Geometry: final body of the model. Coordinates: model frame, mm. A direction names the side the tool comes from. Round coordinates to 2 decimals unless told otherwise and drop trailing zeros. Write each loop counter-clockwise with the first axis right and the second up, starting at its lowest first coordinate (ties: lowest second). Pieces come first, ordered by that corner, then holes. Notation, with made-up numbers: M 33,-24.75 L 81,-24.75 A12 ccw 81,-14.75 Z; hole C -1.75,-10.75 d5. An arc over 180 degrees is marked long. Put each result on its own line as item: value. Start each with the question number.
```python
from build123d import *

# Parameters (mm, degrees)
F0_W      = 80
F0_H      = 17
F0_R      = 1.05
F1_DEPTH  = 2.5
F3_DEPTH  = 43
F5_DEPTH  = 25
F7_D      = 3.3
F8_D      = 3.3
F4_R      = 4.5
F9_DEPTH  = 4.0010001
F10_R     = 4
F11_DEPTH = 10


# Not quite as in the source:
# - a feature names something its author has since deleted; it is built from what else it names


with BuildPart() as f1:
    # F0 (on Top) → F1 (new body, symmetric)
    with BuildSketch(Plane.XY):
        Rectangle(F0_W, F0_H)
        with Locations((-25, 0)):
            Circle(F0_R, mode=Mode.SUBTRACT)
        Circle(F0_R, mode=Mode.SUBTRACT)
        with Locations((25, 0)):
            Circle(F0_R, mode=Mode.SUBTRACT)
    extrude(amount=F1_DEPTH, both=True)

    # F2 (on face) → F3 (join)
    with BuildSketch(Plane.XY.offset(2.5)):
        Polygon((-40, -8.5), (40, -8.5), (40, 8.5), (22, 8.5), (22, -4.5), (-22, -4.5), (-22, 8.5), (-40, 8.5), align=None)
    extrude(amount=F3_DEPTH)

    # F0 (on Top) → F5 (cut)
    with BuildSketch(Plane.XY):
        with Locations((-25, 0)):
            Circle(F0_R)
        Circle(F0_R)
        with Locations((25, 0)):
            Circle(F0_R)
    extrude(amount=F5_DEPTH, mode=Mode.SUBTRACT)

    # F7 (through all)
    with Locations(Plane(origin=(0, 8.5, 0), x_dir=(-1, 0, 0), z_dir=(0, 1, 0))):
        with Locations((25, 0), (-25, 0)):
            Hole(F7_D / 2)

    # F8 (through all)
    with Locations(Plane(origin=(0, -4.5, 0), x_dir=(-1, 0, 0), z_dir=(0, 1, 0))):
        with Locations((15.5, 40), (-15.5, 40), (-15.5, 9), (15.5, 9)):
            Hole(F8_D / 2)

    # F4 (on face) → F9 (cut, through all)
    with BuildSketch(Plane(origin=(0, -4.5, 0), x_dir=(-1, 0, 0), z_dir=(0, 1, 0))):
        with Locations((0, 24.5)):
            Circle(F4_R)
    extrude(amount=-F9_DEPTH, mode=Mode.SUBTRACT)

    # F10 (on face) → F11 (cut)
    with BuildSketch(Plane.XZ.offset(8.5)):
        with Locations((-28, 24.5)):
            Circle(F10_R)
        with Locations((28, 24.5)):
            Circle(F10_R)
    extrude(amount=-F11_DEPTH, mode=Mode.SUBTRACT)


solid = f1.part
```
1) First-contact query: pin 1 (2 mm diameter, centred on x = -15.5, z = 18.5, fed in from +Y); pin 2 (1.3 mm diameter, centred on x = 25, y = 0, fed in from -Z); pin 3 (3 mm diameter, centred on x = -15.5, z = 40, fed in from +Y). Flat tips, straight axial feed; report the tip coordinate or a pass-through.
2) Ray query, probe 1 along Y at (x, z) = (25, 14); probe 2 along X at (y, z) = (3.5, 21); probe 3 along Z at (x, y) = (28, -4). Return the intervals inside material, ascending.
3) Access query for faces 1 (the face through (31.815, -3.57, 25.701)), 2 (the face through (-24.03, -0.4, -2.03)), 3 (the face through (-22, 2, 24)). Directions: +Z, -Z, +X, -X, +Y, -Y. A direction counts if a zero-diameter tool reaches every point of the face in a straight line with its end or side. Return the directions, or none.
4) Section D-D, the plane y = -2. Output: boundary loops of the cut face in (x, z), and give its area (3 significant figures).
5) Section B-B, the plane x = 15.5. Output: boundary loops of the cut face in (y, z).
6) Draft query along X for faces 4 (the face through (40, 0, 21)), 5 (the face through (-1, -8.5, 16)), 6 (the face through (23.95, 0.05, 12.97)). Return one class per face: +X half, -X half, draft (parallel to the pull), parting line (faces both ways), or undercut.
7) Section C-C, the plane z = 0. Output: boundary loops of the cut face in (x, y), and give its area (3 significant figures).
8) Section A-A, the plane z = 9. Output: boundary loops of the cut face in (x, y).
Solved:
1. pin 1: stops at y = -4.5
1. pin 2: stops at z = 26.14
1. pin 3: passes through
2. probe 1: y = -8.5 to -1.05, 1.05 to 8.5
2. probe 2: x = -40 to -22, 22 to 40
2. probe 3: z = -2.5 to 20.5, 28.5 to 45.5
3. face 1: -Y
3. face 2: -Z
3. face 3: +Z, +Y
4. outline: M -40,-2.5 L 40,-2.5 L 40,45.5 L 22,45.5 L 22,2.5 L -22,2.5 L -22,45.5 L -40,45.5 Z; hole C -28,24.5 d8; hole C -25,0 d3.3; hole C 25,0 d3.3; hole C 28,24.5 d8
4. area: 1,830 mm2
5. outline: M -8.5,-2.5 L 8.5,-2.5 L 8.5,2.5 L -4.5,2.5 L -4.5,7.35 L -8.5,7.35 Z; M -8.5,10.65 L -4.5,10.65 L -4.5,38.35 L -8.5,38.35 Z; M -8.5,41.65 L -4.5,41.65 L -4.5,45.5 L -8.5,45.5 Z
6. face 4: +X half
6. face 5: draft
6. face 6: undercut
7. outline: M -40,-8.5 L -26.65,-8.5 L -26.65,8.5 L -40,8.5 Z; M -23.35,-8.5 L 23.35,-8.5 L 23.35,8.5 L -23.35,8.5 Z; M 26.65,-8.5 L 40,-8.5 L 40,8.5 L 26.65,8.5 Z; hole C 0,0 d2.1
7. area: 1,240 mm2
8. outline: M -40,-8.5 L -17.15,-8.5 L -17.15,-4.5 L -22,-4.5 L -22,8.5 L -40,8.5 Z; M -13.85,-8.5 L 13.85,-8.5 L 13.85,-4.5 L -13.85,-4.5 Z; M 17.15,-8.5 L 40,-8.5 L 40,8.5 L 22,8.5 L 22,-4.5 L 17.15,-4.5 Z; hole C -25,0 d2.1; hole C 25,0 d2.1
